from build123d import *

# Parameters (mm, degrees)
BOSS_EXTRUDE1_DEPTH = 15
CHAMFER1_SIZE       = 5
SKETCH3_W           = 10
SKETCH3_H           = 10
CUT_EXTRUDE1_DEPTH  = 24
CHAMFER2_SIZE       = 2.5
SKETCH4_W           = 3
SKETCH4_H           = 3
CUT_EXTRUDE2_DEPTH  = 3.535533906


with BuildPart() as part:
    # Sketch1 → Boss-Extrude1 (new body)
    with BuildSketch(Plane(origin=(0, 0, 0), x_dir=(1, 0, 0), z_dir=(0, 1, 0))):
        Polygon((-48.5, 13.5), (51.5, 13.5), (51.5, -11.5), (48.5, -11.5), (48.5, 11.5), (-48.5, 11.5), align=None)
    extrude(amount=BOSS_EXTRUDE1_DEPTH)

    # Chamfer1
    chamfer1_edges = [part.edges().sort_by_distance(p)[0] for p in [
        (51.5, 7.5, -13.5),
        (48.5, 7.5, -11.5),
    ]]
    chamfer(chamfer1_edges, length=CHAMFER1_SIZE)

    # Sketch3 → Cut-Extrude1 (cut)
    with BuildSketch(Plane(origin=(51.5, 0, 0), x_dir=(0, 0, -1), z_dir=(1, 0, 0))):
        with Locations((-6.5, 7.5)):
            Rectangle(SKETCH3_W, SKETCH3_H)
    extrude(amount=-CUT_EXTRUDE1_DEPTH, mode=Mode.SUBTRACT)

    # Chamfer2
    # the kernel refuses this chamfer: 2.5 mm, written as the material it takes off along each edge
    with BuildSketch(Plane(origin=(-48.5, -6.42920747, -13.5), x_dir=(0.9996219169112968, 0, -0.027495876610586282), z_dir=(0, 1, 0))) as chamfer2_piece_1:
        Polygon((CHAMFER2_SIZE * 0.999621916911, -CHAMFER2_SIZE * 0.0274958766106), (-CHAMFER2_SIZE * 0.0274958766106, -CHAMFER2_SIZE * 0.999621916911), (0, 0), align=None)
    extrude(amount=27.85841494, mode=Mode.SUBTRACT)

    # Sketch4 → Cut-Extrude2 (cut)
    with BuildSketch(Plane(origin=(30, 0, -30), x_dir=(-0.7071067811865442, 0, -0.7071067811865509), z_dir=(0.7071067811865509, 0, -0.7071067811865442))):
        with Locations((-26.870057685, 1.5)):
            Rectangle(SKETCH4_W, SKETCH4_H)
        with Locations((-26.870057685, 13.5)):
            Rectangle(SKETCH4_W, SKETCH4_H)
    extrude(amount=-CUT_EXTRUDE2_DEPTH, mode=Mode.SUBTRACT)


solid = part.part
Here's how the part is built. I have some questions about the finished solid (model axes, mm). A direction names the side the tool comes from. Round coordinates to 2 decimals unless told otherwise and drop trailing zeros. Write each loop counter-clockwise with the first axis right and the second up, starting at its lowest first coordinate (ties: lowest second). Pieces come first, ordered by that corner, then holes. Notation, with made-up numbers: (-36.75, 24.25) -> (6.25, 24.25) arc R21 cw to (6.25, 47.25) -> close; hole circle Ø3 at (79.5, -8.75). An arc over 180 degrees is marked (long way). One line per item, written item: value.
1) Suppose I cut it at C-C on y = 7. List the corners of the cut face in (x, z) for me.
Filled sheet:
outline: (-48, -11.5) -> (-46, -13.5) -> (46.5, -13.5) -> (51.5, -8.5) -> (51.5, 1.5) -> (48.5, 1.5) -> (48.5, -6.5) -> (43.5, -11.5) -> close
2) Suppose I cut it at A-A on y = 13.5. List the corners of the cut face in (x, z) for me, plus the area to 3 significant figures.
Filled sheet:
outline: (-48, -11.5) -> (-46, -13.5) -> (46.5, -13.5) -> (47.94, -12.06) -> (45.44, -9.56) -> (43.5, -11.5) -> close; (47.56, -7.44) -> (50.06, -9.94) -> (51.5, -8.5) -> (51.5, 11.5) -> (48.5, 11.5) -> (48.5, -6.5) -> close
area: 255 mm2
3) If I drill on line 1 (X direction, y = 11.5, z = -5); line 2 (Z direction, x = 15, y = 5.75); line 3 (X direction, y = 4.25, z = -6.75), over which ranges is the centre line in solid material (lowest first)? Write a range as [from, to].
Filled sheet:
line 1: x = [48.5, 51.5]
line 2: z = [-13.5, -11.5]
line 3: x = [48.25, 51.5]
4) I'm going to push flat-ended pins straight in: pin 1 Ø3 at (y, z) = (6, -0.5) entering from -X; pin 2 Ø0.9 at (x, y) = (50.5, 6) entering from +Z; pin 3 Ø6 at (x, y) = (38.5, 12) entering from +Z. Where does each tip first touch, or does it pass through?
Filled sheet:
pin 1: stops at x = 48.5
pin 2: stops at z = 1.5
pin 3: stops at z = -11.5
5) For faces 1 (the face through (48, 12, -10)), 2 (the face through (50, 0, 1)), 3 (the face through (50, 2.5, 7)), which set-ups out of +Z, -Z, +X, -X, +Y, -Y let a thin tool reach every point of the face, with its end or its side?
Filled sheet:
face 1: +Y
face 2: +Z, -Z, +X, -X, -Y
face 3: +Z, +X, -X
6) We'd pull the mould along Z, two halves only. Please class faces 4 (the face through (48, 3, -10)), 5 (the face through (1, 0, -12)), 6 (the face through (50, 1, 11.5)), 7 (the face through (-47, 7.4, -12.5)): released by +Z, released by -Z, zero draft, split by the parting line, or undercut.
Filled sheet:
face 4: undercut
face 5: zero draft
face 6: released by +Z
face 7: released by -Z
7) Suppose I cut it at B-B on z = 9.5. List the corners of the cut face in (x, y) for me, plus the area to 3 significant figures.
Filled sheet:
outline: (48.5, 0) -> (51.5, 0) -> (51.5, 2.5) -> (48.5, 2.5) -> close; (48.5, 12.5) -> (51.5, 12.5) -> (51.5, 15) -> (48.5, 15) -> close
area: 15.0 mm2
8) Suppose I cut it at D-D on z = -0.5. List the corners of the cut face in (x, y) for me, plus the area to 3 significant figures.
Filled sheet:
outline: (48.5, 0) -> (51.5, 0) -> (51.5, 15) -> (48.5, 15) -> close
area: 45.0 mm2
